Check sheet for the modelled part. Datum: model origin and axes. Units: mm. Face numbers are marked on the shaded views. A direction names the side the tool comes from. Round coordinates to 2 decimals unless told otherwise and drop trailing zeros. Write each loop counter-clockwise with the first axis right and the second up, starting at its lowest first coordinate (ties: lowest second). Pieces come first, ordered by that corner, then holes.
Item 1: Section check D-D, the plane x = -28. State how many separate pieces and enclosed holes the cut face has, plus the area to 3 significant figures.
Item 2: Section check C-C, the plane z = 53. Record the cut outline in (x, y), plus the area to 3 significant figures.
Item 3: Set-up check for the marked faces 1, 2 and 3: record each of +Z, -Z, +X, -X, +Y, -Y from which the full face is reachable in a straight line by a thin tool's end or side.
Item 4: Depth check by flat-ended pin: pin 1 (2 mm diameter, centred on x = -44.5, z = 40, fed in from -Y); pin 2 (2.5 mm diameter, centred on x = -5, y = -77, fed in from -Z); pin 3 (2.5 mm diameter, centred on x = -35.5, z = 48, fed in from +Y). Enter the tip coordinate at first touch or a pass-through.
Item 5: Material ranges on line 1 along X through (y, z) = (-19.5, 3); line 2 along X through (y, z) = (-77, 3); line 3 along Z through (x, y) = (-9, -78), recorded low to high.
Item 6: Section check A-A, the plane y = -107. Record the cut outline in (x, z).
Item 7: Section check B-B, the plane x = -45.5. Record the cut outline in (y, z), plus the area to 3 significant figures.
Item 8: Release check for a two-part mould opening along Z. For the marked faces 4, 5 and 6 record: pulls with the +Z half, pulls with the -Z half, needs draft (parallel to the pull), parting line crosses it, or undercut.
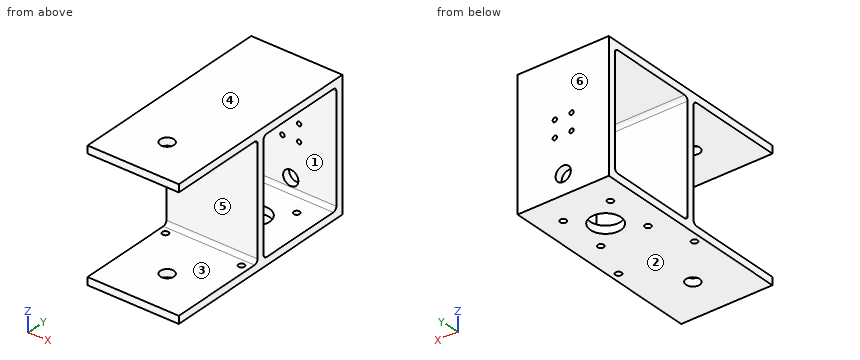
from build123d import *

# Parameters (mm, degrees)
BOSS_EXTRUDE1_DEPTH = 60
SKETCH2_W           = 75
SKETCH2_H           = 60
CUT_EXTRUDE1_DEPTH  = 60
CUT_EXTRUDE2_REACH  = 137
SKETCH3_R           = 1.425
SKETCH3_R_2         = 5
CUT_EXTRUDE3_REACH  = 87
SKETCH4_R           = 4.5
SKETCH4_R_2         = 10
SKETCH4_R_3         = 2
FILLET1_R           = 2.5
FILLET2_R           = 2.5
FILLET3_R           = 2.5
FILLET4_R           = 2.5
FILLET5_R           = 2.5
FILLET6_R           = 2.5
CUT_EXTRUDE4_REACH  = 87
SKETCH5_R           = 4.5


with BuildPart() as part:
    # Sketch1 → Boss-Extrude1 (new body)
    with BuildSketch(Plane(origin=(0, 0, 0), x_dir=(0, 0, -1), z_dir=(1, 0, 0))):
        Polygon((0, 0), (0, -135), (-5, -135), (-5, -70), (-80, -70), (-80, -135), (-85, -135), (-85, 0), align=None)
    extrude(amount=-BOSS_EXTRUDE1_DEPTH)

    # Sketch2 → Cut-Extrude1 (cut)
    with BuildSketch(Plane(origin=(0, 0, 0), x_dir=(0, 0, -1), z_dir=(1, 0, 0))):
        with Locations((-42.5, -35)):
            Rectangle(SKETCH2_W, SKETCH2_H)
    extrude(amount=-CUT_EXTRUDE1_DEPTH, mode=Mode.SUBTRACT)

    # Sketch3 → Cut-Extrude2 (cut, up to next)
    with BuildSketch(Plane(origin=(0, 0, 0), x_dir=(1, 0, 0), z_dir=(0, 1, 0)), mode=Mode.PRIVATE) as cut_extrude2_sk1:
        with Locations((-35.5, -37)):
            Circle(SKETCH3_R)
    cut_extrude2_tool1 = extrude(cut_extrude2_sk1.sketch, amount=-CUT_EXTRUDE2_REACH, mode=Mode.PRIVATE) & part.part
    add(cut_extrude2_tool1.solids().sort_by_distance((-35.5, 0, 37))[0], mode=Mode.SUBTRACT)
    # Sketch3 → Cut-Extrude2 (cut, up to next)
    with BuildSketch(Plane(origin=(0, 0, 0), x_dir=(1, 0, 0), z_dir=(0, 1, 0)), mode=Mode.PRIVATE) as cut_extrude2_sk2:
        with Locations((-24.5, -37)):
            Circle(SKETCH3_R)
    cut_extrude2_tool2 = extrude(cut_extrude2_sk2.sketch, amount=-CUT_EXTRUDE2_REACH, mode=Mode.PRIVATE) & part.part
    add(cut_extrude2_tool2.solids().sort_by_distance((-24.5, 0, 37))[0], mode=Mode.SUBTRACT)
    # Sketch3 → Cut-Extrude2 (cut, up to next)
    with BuildSketch(Plane(origin=(0, 0, 0), x_dir=(1, 0, 0), z_dir=(0, 1, 0)), mode=Mode.PRIVATE) as cut_extrude2_sk3:
        with Locations((-24.5, -48)):
            Circle(SKETCH3_R)
    cut_extrude2_tool3 = extrude(cut_extrude2_sk3.sketch, amount=-CUT_EXTRUDE2_REACH, mode=Mode.PRIVATE) & part.part
    add(cut_extrude2_tool3.solids().sort_by_distance((-24.5, 0, 48))[0], mode=Mode.SUBTRACT)
    # Sketch3 → Cut-Extrude2 (cut, up to next)
    with BuildSketch(Plane(origin=(0, 0, 0), x_dir=(1, 0, 0), z_dir=(0, 1, 0)), mode=Mode.PRIVATE) as cut_extrude2_sk4:
        with Locations((-35.5, -48)):
            Circle(SKETCH3_R)
    cut_extrude2_tool4 = extrude(cut_extrude2_sk4.sketch, amount=-CUT_EXTRUDE2_REACH, mode=Mode.PRIVATE) & part.part
    add(cut_extrude2_tool4.solids().sort_by_distance((-35.5, 0, 48))[0], mode=Mode.SUBTRACT)
    # Sketch3 → Cut-Extrude2 (cut, up to next)
    with BuildSketch(Plane(origin=(0, 0, 0), x_dir=(1, 0, 0), z_dir=(0, 1, 0)), mode=Mode.PRIVATE) as cut_extrude2_sk5:
        with Locations((-30, -13)):
            Circle(SKETCH3_R_2)
    cut_extrude2_tool5 = extrude(cut_extrude2_sk5.sketch, amount=-CUT_EXTRUDE2_REACH, mode=Mode.PRIVATE) & part.part
    add(cut_extrude2_tool5.solids().sort_by_distance((-30, 0, 13))[0], mode=Mode.SUBTRACT)

    # Sketch4 → Cut-Extrude3 (cut, up to next)
    with BuildSketch(Plane.XY, mode=Mode.PRIVATE) as cut_extrude3_sk1:
        with Locations((-30, -107)):
            Circle(SKETCH4_R)
    cut_extrude3_tool1 = extrude(cut_extrude3_sk1.sketch, amount=CUT_EXTRUDE3_REACH, mode=Mode.PRIVATE) & part.part
    add(cut_extrude3_tool1.solids().sort_by_distance((-30, -107, 0))[0], mode=Mode.SUBTRACT)
    # Sketch4 → Cut-Extrude3 (cut, up to next)
    with BuildSketch(Plane.XY, mode=Mode.PRIVATE) as cut_extrude3_sk2:
        with Locations((-30, -35)):
            Circle(SKETCH4_R_2)
    cut_extrude3_tool2 = extrude(cut_extrude3_sk2.sketch, amount=CUT_EXTRUDE3_REACH, mode=Mode.PRIVATE) & part.part
    add(cut_extrude3_tool2.solids().sort_by_distance((-30, -35, 0))[0], mode=Mode.SUBTRACT)
    # Sketch4 → Cut-Extrude3 (cut, up to next)
    with BuildSketch(Plane.XY, mode=Mode.PRIVATE) as cut_extrude3_sk3:
        with Locations((-5, -77)):
            Circle(SKETCH4_R_3)
    cut_extrude3_tool3 = extrude(cut_extrude3_sk3.sketch, amount=CUT_EXTRUDE3_REACH, mode=Mode.PRIVATE) & part.part
    add(cut_extrude3_tool3.solids().sort_by_distance((-5, -77, 0))[0], mode=Mode.SUBTRACT)
    # Sketch4 → Cut-Extrude3 (cut, up to next)
    with BuildSketch(Plane.XY, mode=Mode.PRIVATE) as cut_extrude3_sk4:
        with Locations((-55, -77)):
            Circle(SKETCH4_R_3)
    cut_extrude3_tool4 = extrude(cut_extrude3_sk4.sketch, amount=CUT_EXTRUDE3_REACH, mode=Mode.PRIVATE) & part.part
    add(cut_extrude3_tool4.solids().sort_by_distance((-55, -77, 0))[0], mode=Mode.SUBTRACT)
    # Sketch4 → Cut-Extrude3 (cut, up to next)
    with BuildSketch(Plane.XY, mode=Mode.PRIVATE) as cut_extrude3_sk5:
        with Locations((-14.5, -19.5)):
            Circle(SKETCH4_R_3)
    cut_extrude3_tool5 = extrude(cut_extrude3_sk5.sketch, amount=CUT_EXTRUDE3_REACH, mode=Mode.PRIVATE) & part.part
    add(cut_extrude3_tool5.solids().sort_by_distance((-14.5, -19.5, 0))[0], mode=Mode.SUBTRACT)
    # Sketch4 → Cut-Extrude3 (cut, up to next)
    with BuildSketch(Plane.XY, mode=Mode.PRIVATE) as cut_extrude3_sk6:
        with Locations((-45.5, -19.5)):
            Circle(SKETCH4_R_3)
    cut_extrude3_tool6 = extrude(cut_extrude3_sk6.sketch, amount=CUT_EXTRUDE3_REACH, mode=Mode.PRIVATE) & part.part
    add(cut_extrude3_tool6.solids().sort_by_distance((-45.5, -19.5, 0))[0], mode=Mode.SUBTRACT)
    # Sketch4 → Cut-Extrude3 (cut, up to next)
    with BuildSketch(Plane.XY, mode=Mode.PRIVATE) as cut_extrude3_sk7:
        with Locations((-45.5, -50.5)):
            Circle(SKETCH4_R_3)
    cut_extrude3_tool7 = extrude(cut_extrude3_sk7.sketch, amount=CUT_EXTRUDE3_REACH, mode=Mode.PRIVATE) & part.part
    add(cut_extrude3_tool7.solids().sort_by_distance((-45.5, -50.5, 0))[0], mode=Mode.SUBTRACT)
    # Sketch4 → Cut-Extrude3 (cut, up to next)
    with BuildSketch(Plane.XY, mode=Mode.PRIVATE) as cut_extrude3_sk8:
        with Locations((-14.5, -50.5)):
            Circle(SKETCH4_R_3)
    cut_extrude3_tool8 = extrude(cut_extrude3_sk8.sketch, amount=CUT_EXTRUDE3_REACH, mode=Mode.PRIVATE) & part.part
    add(cut_extrude3_tool8.solids().sort_by_distance((-14.5, -50.5, 0))[0], mode=Mode.SUBTRACT)

    # Fillet1
    fillet1_edges = [part.edges().sort_by_distance(p)[0] for p in [
        (-30, -70, 80),
    ]]
    fillet(fillet1_edges, radius=FILLET1_R)

    # Fillet2
    fillet2_edges = [part.edges().sort_by_distance(p)[0] for p in [
        (-30, -70, 5),
    ]]
    fillet(fillet2_edges, radius=FILLET2_R)

    # Fillet3
    fillet3_edges = [part.edges().sort_by_distance(p)[0] for p in [
        (-30, -65, 80),
    ]]
    fillet(fillet3_edges, radius=FILLET3_R)

    # Fillet4
    fillet4_edges = [part.edges().sort_by_distance(p)[0] for p in [
        (-30, -65, 5),
    ]]
    fillet(fillet4_edges, radius=FILLET4_R)

    # Fillet5
    fillet5_edges = [part.edges().sort_by_distance(p)[0] for p in [
        (-30, -5, 5),
    ]]
    fillet(fillet5_edges, radius=FILLET5_R)

    # Fillet6
    fillet6_edges = [part.edges().sort_by_distance(p)[0] for p in [
        (-30, -5, 80),
    ]]
    fillet(fillet6_edges, radius=FILLET6_R)

    # Sketch5 → Cut-Extrude4 (cut, up to next)
    with BuildSketch(Plane.XY.offset(85), mode=Mode.PRIVATE) as cut_extrude4_sk1:
        with Locations((-30, -107)):
            Circle(SKETCH5_R)
    cut_extrude4_tool1 = extrude(cut_extrude4_sk1.sketch, amount=-CUT_EXTRUDE4_REACH, mode=Mode.PRIVATE) & part.part
    add(cut_extrude4_tool1.solids().sort_by_distance((-30, -107, 85))[0], mode=Mode.SUBTRACT)


solid = part.part
Values found:
1. separate pieces: 4
1. enclosed holes: 0
1. area: 1,880 mm2
2. outline: (-60, -70) - (0, -70) - (0, -65) - (-60, -65) - close; (-60, -5) - (0, -5) - (0, 0) - (-60, 0) - close
2. area: 600 mm2
3. face 1: +X, -X
3. face 2: -Z, +X, -X, +Y, -Y
3. face 3: +X, -X, -Y
4. pin 1: stops at y = -70
4. pin 2: stops at z = 80
4. pin 3: stops at y = -65
5. line 1: x = -60 to -47.5, -43.5 to -16.5, -12.5 to 0
5. line 2: x = -60 to -57, -53 to -7, -3 to 0
5. line 3: z = 0 to 5, 80 to 85
6. outline: (-60, 0) - (-34.5, 0) - (-34.5, 5) - (-60, 5) - close; (-60, 80) - (-34.5, 80) - (-34.5, 85) - (-60, 85) - close; (-25.5, 0) - (0, 0) - (0, 5) - (-25.5, 5) - close; (-25.5, 80) - (0, 80) - (0, 85) - (-25.5, 85) - close
7. outline: (-135, 0) - (-52.5, 0) - (-52.5, 5) - (-62.5, 5) arc R2.5 cw to (-65, 7.5) - (-65, 77.5) arc R2.5 cw to (-62.5, 80) - (-7.5, 80) arc R2.5 cw to (-5, 77.5) - (-5, 7.5) arc R2.5 cw to (-7.5, 5) - (-17.5, 5) - (-17.5, 0) - (0, 0) - (0, 85) - (-135, 85) - (-135, 80) - (-72.5, 80) arc R2.5 cw to (-70, 77.5) - (-70, 7.5) arc R2.5 cw to (-72.5, 5) - (-135, 5) - close; (-48.5, 0) - (-21.5, 0) - (-21.5, 5) - (-48.5, 5) - close
7. area: 2,070 mm2
8. face 4: pulls with the +Z half
8. face 5: undercut
8. face 6: needs draft
